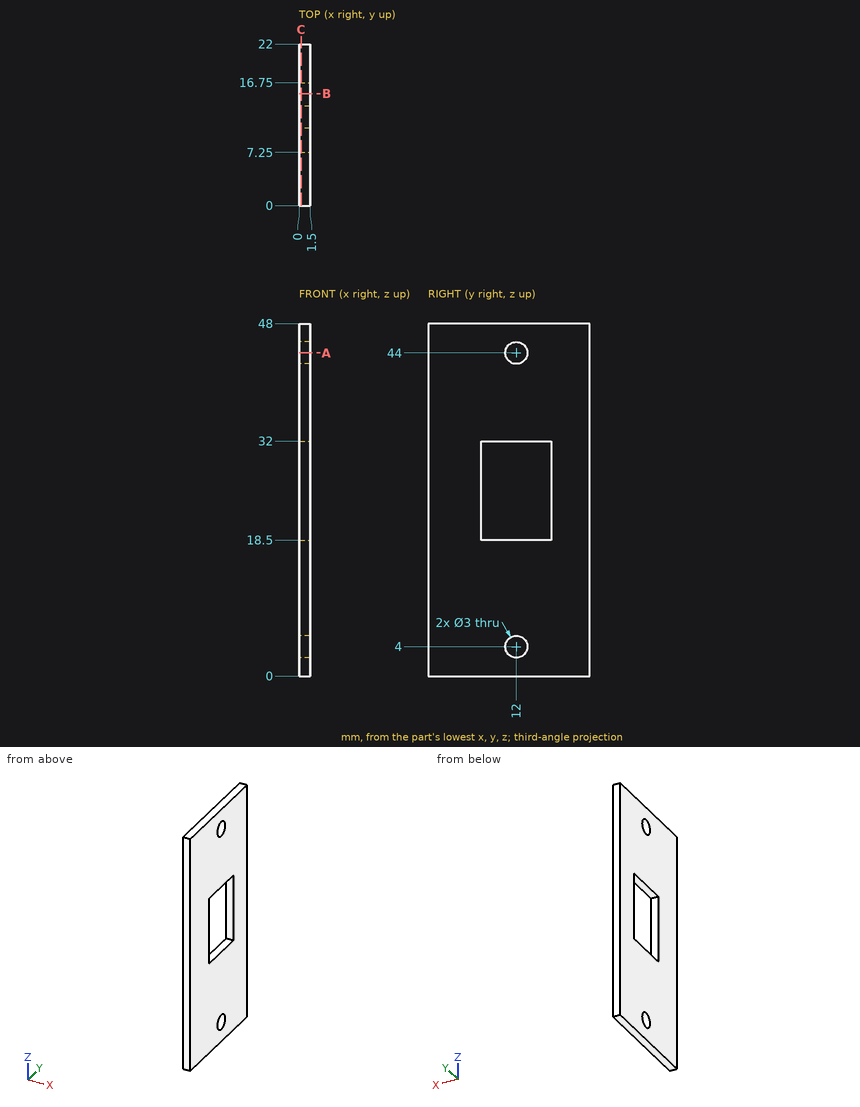
Source: three-view drawing plus pictorial views. Frame: mm from the lowest corner of the part. Round coordinates to 2 decimals unless told otherwise and drop trailing zeros. Write each loop counter-clockwise with the first axis right and the second up, starting at its lowest first coordinate (ties: lowest second). Pieces come first, ordered by that corner, then holes. Notation, with made-up numbers: M 64.25,69.25 L 80.25,69.25 A22 ccw 80.25,99.25 Z; hole C -39,39.25 d1. An arc over 180 degrees is marked long. Write each question's results on one line, items separated by ' | '.
Q1. Section query C-C (x = 0.25). Return loops of the section in (y, z).
Results:
outline: M 0,0 L 22,0 L 22,48 L 0,48 Z; hole M 7.25,18.5 L 16.75,18.5 L 16.75,32 L 7.25,32 Z; hole C 12,4 d3; hole C 12,44 d3
Q2. Line query: line 1 along Z through (x, y) = (0.9, 12); line 2 along Y through (x, z) = (0.85, 44); line 3 along Y through (x, z) = (1, 19). Output: solid intervals per line, ascending.
Results:
line 1: z = 0 to 2.5, 5.5 to 18.5, 32 to 42.5, 45.5 to 48 | line 2: y = 0 to 10.5, 13.5 to 22 | line 3: y = 0 to 7.25, 16.75 to 22
Q3. Section query A-A (z = 44). Return loops of the section in (x, y), and give its area (3 significant figures).
Results:
outline: M 0,0 L 1.5,0 L 1.5,10.5 L 0,10.5 Z; M 0,13.5 L 1.5,13.5 L 1.5,22 L 0,22 Z | area: 28.5 mm^2
Q4. Pin query (flat end, axial travel): P1, Ø2.5, axis at y = 12, z = 4, coming from the +X side. Return the tip coordinate at first contact, or that it passes through.
Results:
P1: passes through
Q5. Section query B-B (y = 15.25). Return loops of the section in (x, z).
Results:
outline: M 0,0 L 1.5,0 L 1.5,18.5 L 0,18.5 Z; M 0,32 L 1.5,32 L 1.5,48 L 0,48 Z
